```python
from build123d import *

# Parameters (mm, degrees)
F1_DEPTH = 1
F2_DEPTH = 2


with BuildPart() as f1:
    # F0 (on Top) → F1 (new body)
    with BuildSketch(Plane.XY):
        with BuildLine():
            Line((25, 15), (-25, 15))
            ThreePointArc((-25, 15), (-28.5355339059, 13.5355339059), (-30, 10))
            Line((-30, 10), (-30, -10))
            ThreePointArc((-30, -10), (-28.5355339059, -13.5355339059), (-25, -15))
            Line((-25, -15), (25, -15))
            ThreePointArc((25, -15), (28.5355339059, -13.5355339059), (30, -10))
            Line((30, -10), (30, 10))
            ThreePointArc((30, 10), (28.5355339059, 13.5355339059), (25, 15))
        make_face()
        with BuildLine():
            Line((-27.5, 12.0571891388), (-27.5, 12.5))
            Line((-27.5, 12.5), (-27.0571891388, 12.5))
            ThreePointArc((-27.0571891388, 12.5), (-25.517766953, 13.4270717335), (-23.75, 13.75))
            Line((-23.75, 13.75), (23.75, 13.75))
            ThreePointArc((23.75, 13.75), (25.517766953, 13.4270717335), (27.0571891388, 12.5))
            Line((27.0571891388, 12.5), (27.5, 12.5))
            Line((27.5, 12.5), (27.5, 12.0571891388))
            ThreePointArc((27.5, 12.0571891388), (28.4270717335, 10.517766953), (28.75, 8.75))
            Line((28.75, 8.75), (28.75, -8.75))
            ThreePointArc((28.75, -8.75), (28.4270717335, -10.517766953), (27.5, -12.0571891388))
            Line((27.5, -12.0571891388), (27.5, -12.5))
            Line((27.5, -12.5), (27.0571891388, -12.5))
            ThreePointArc((27.0571891388, -12.5), (25.517766953, -13.4270717335), (23.75, -13.75))
            Line((23.75, -13.75), (-23.75, -13.75))
            ThreePointArc((-23.75, -13.75), (-25.517766953, -13.4270717335), (-27.0571891388, -12.5))
            Line((-27.0571891388, -12.5), (-27.5, -12.5))
            Line((-27.5, -12.5), (-27.5, -12.0571891388))
            ThreePointArc((-27.5, -12.0571891388), (-28.4270717335, -10.517766953), (-28.75, -8.75))
            Line((-28.75, -8.75), (-28.75, 8.75))
            ThreePointArc((-28.75, 8.75), (-28.4270717335, 10.517766953), (-27.5, 12.0571891388))
        make_face(mode=Mode.SUBTRACT)
    extrude(amount=F1_DEPTH)

    # F0 (on Top) → F2 (join)
    with BuildSketch(Plane.XY):
        with BuildLine():
            Line((27.0571891388, 12.5), (-27.0571891388, 12.5))
            ThreePointArc((-27.0571891388, 12.5), (-27.2855339059, 12.2855339059), (-27.5, 12.0571891388))
            Line((-27.5, 12.0571891388), (-27.5, -12.0571891388))
            ThreePointArc((-27.5, -12.0571891388), (-27.2855339059, -12.2855339059), (-27.0571891388, -12.5))
            Line((-27.0571891388, -12.5), (27.0571891388, -12.5))
            ThreePointArc((27.0571891388, -12.5), (27.2855339059, -12.2855339059), (27.5, -12.0571891388))
            Line((27.5, -12.0571891388), (27.5, 12.0571891388))
            ThreePointArc((27.5, 12.0571891388), (27.2855339059, 12.2855339059), (27.0571891388, 12.5))
        make_face()
        with BuildLine():
            ThreePointArc((28.75, 8.75), (28.4270717335, 10.517766953), (27.5, 12.0571891388))
            Line((27.5, 12.0571891388), (27.5, -12.0571891388))
            ThreePointArc((27.5, -12.0571891388), (28.4270717335, -10.517766953), (28.75, -8.75))
            Line((28.75, -8.75), (28.75, 8.75))
        make_face()
        with BuildLine():
            ThreePointArc((-23.75, 13.75), (-25.517766953, 13.4270717335), (-27.0571891388, 12.5))
            Line((-27.0571891388, 12.5), (27.0571891388, 12.5))
            ThreePointArc((27.0571891388, 12.5), (25.517766953, 13.4270717335), (23.75, 13.75))
            Line((23.75, 13.75), (-23.75, 13.75))
        make_face()
        with BuildLine():
            Line((27.0571891388, -12.5), (-27.0571891388, -12.5))
            ThreePointArc((-27.0571891388, -12.5), (-25.517766953, -13.4270717335), (-23.75, -13.75))
            Line((-23.75, -13.75), (23.75, -13.75))
            ThreePointArc((23.75, -13.75), (25.517766953, -13.4270717335), (27.0571891388, -12.5))
        make_face()
        with BuildLine():
            Line((-27.5, -12.0571891388), (-27.5, 12.0571891388))
            ThreePointArc((-27.5, 12.0571891388), (-28.4270717335, 10.517766953), (-28.75, 8.75))
            Line((-28.75, 8.75), (-28.75, -8.75))
            ThreePointArc((-28.75, -8.75), (-28.4270717335, -10.517766953), (-27.5, -12.0571891388))
        make_face()
    extrude(amount=F2_DEPTH)


solid = f1.part
```
Build history of the part. All positions in model axes, mm. Give positions to 0.01 mm unless a question says otherwise; leave off trailing zeros. Loops run counter-clockwise (first coordinate to the right, second up) from the corner with the lowest first, then second, coordinate; pieces in that order, holes last. Notation, with made-up numbers: (-19, -27) - (20, -27) arc R30 cw to (20, -1) - close; hole circle Ø8 at (11, 83). An arc over 180 degrees is marked (long way). Use a Markdown table: item, result.
(1) Band-saw the part on B-B (z = 1.65). Give the cut face in (x, y), and give its area (3 significant figures).
Taken from the geometry:
| item | result |
|---|---|
| outline | (-28.75, -8.75) arc R5 ccw to (-23.75, -13.75) - (23.75, -13.75) arc R5 ccw to (28.75, -8.75) - (28.75, 8.75) arc R5 ccw to (23.75, 13.75) - (-23.75, 13.75) arc R5 ccw to (-28.75, 8.75) - close |
| area | 1,560 mm2 |
(2) Band-saw the part on A-A (y = -5.5). Give the cut face in (x, z).
Taken from the geometry:
| item | result |
|---|---|
| outline | (-30, 0) - (30, 0) - (30, 1) - (28.75, 1) - (28.75, 2) - (-28.75, 2) - (-28.75, 1) - (-30, 1) - close |
(3) Drop flat-ended pins along their axis: pin 1 Ø0.5 at (x, z) = (-7, 1.5) entering from +Y; pin 2 Ø0.5 at (x, z) = (-27, 0.5) entering from +Y; pin 3 Ø0.5 at (y, z) = (12.5, 0.5) entering from +X. Give the stop position or say it passes through.
Taken from the geometry:
| item | result |
|---|---|
| pin 1 | y = 13.75 |
| pin 2 | y = 14.68 |
| pin 3 | x = 29.47 |
(4) Band-saw the part on C-C (x = 18.5). Give the cut face in (y, z).
Taken from the geometry:
| item | result |
|---|---|
| outline | (-15, 0) - (15, 0) - (15, 1) - (13.75, 1) - (13.75, 2) - (-13.75, 2) - (-13.75, 1) - (-15, 1) - close |
(5) Wall check: line 1 along Y through (x, z) = (-8.5, 1.8); line 2 along X through (y, z) = (5.75, 1.15); line 3 along X through (y, z) = (-12.25, 1.9). Give the ranges that are in metal, low to high.
Taken from the geometry:
| item | result |
|---|---|
| line 1 | -13.75 to 13.75 |
| line 2 | -28.75 to 28.75 |
| line 3 | -27.32 to 27.32 |
